For this review, use the dimensioned drawing (mm, ordinates from the lowest corner) and the shaded views. Round coordinates to 2 decimals unless told otherwise and drop trailing zeros. Loops run counter-clockwise (first coordinate to the right, second up) from the corner with the lowest first, then second, coordinate; pieces in that order, holes last.
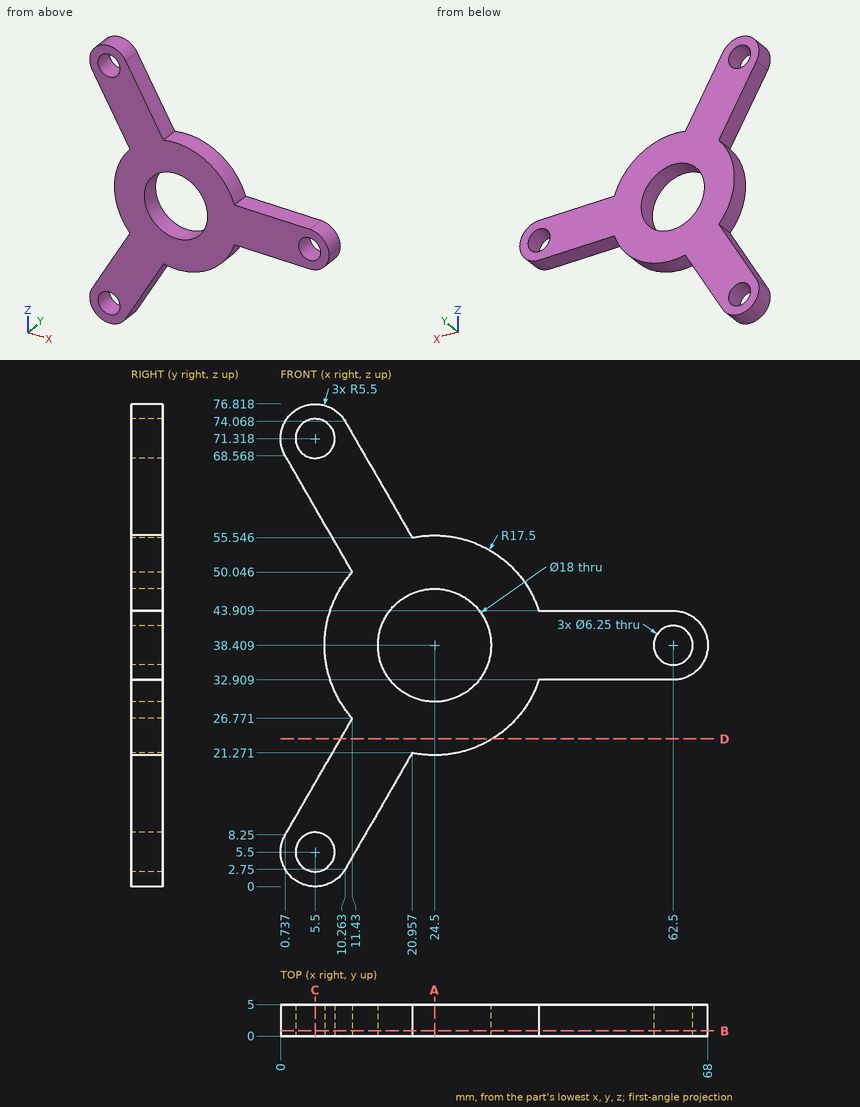
(1) Add section A-A (x = 24.5). Give the boundary of the cut face in (y, z).
(2) Add section C-C (x = 5.5). Give the boundary of the cut face in (y, z) (1 decimal).
(3) Add section D-D (z = 23.5). Give the boundary of the cut face in (x, y).
(4) Add section B-B (y = 0.8). Give the number of separate pieces and of enclosed holes in the cut face, plus the area to 3 significant figures.
(5) Insertion check: pin 1 Ø2 at (y, z) = (2, 63.5) entering from +X; pin 2 Ø2.5 at (x, y) = (50.5, 3) entering from +Z; pin 3 Ø1.5 at (x, y) = (52.5, 3.5) entering from -Z. Each pin has a flat end and moves straight along its axis. Give the tip position at first contact, or say it passes through.
(6) For L1, parallel to Z at x = 5.5, y = 2.25 (1 decimal); L2, parallel to Z at x = 9, y = 1.4 (1 decimal); L3, parallel to Z at x = 43.5, y = 4.35, list the stretches that pass through material, from the lowest coordinate up.
Outcome:
1. outline: (0, 20.91) - (5, 20.91) - (5, 29.41) - (0, 29.41) - close; (0, 47.41) - (5, 47.41) - (5, 55.91) - (0, 55.91) - close
2. outline: (0, 0) - (5, 0) - (5, 2.4) - (0, 2.4) - close; (0, 8.6) - (5, 8.6) - (5, 16.5) - (0, 16.5) - close; (0, 60.3) - (5, 60.3) - (5, 68.2) - (0, 68.2) - close; (0, 74.4) - (5, 74.4) - (5, 76.8) - (0, 76.8) - close
3. outline: (9.54, 0) - (33.66, 0) - (33.66, 5) - (9.54, 5) - close
4. separate pieces: 1
4. enclosed holes: 4
4. area: 1,440 mm2
5. pin 1: stops at x = 16.94
5. pin 2: stops at z = 43.91
5. pin 3: stops at z = 32.91
6. L1: z = 0 to 2.4, 8.6 to 16.5, 60.3 to 68.2, 74.4 to 76.8
6. L2: z = 1.3 to 22.6, 30.3 to 46.5, 54.3 to 75.6
6. L3: z = 32.91 to 43.91
